from build123d import *

# Parameters (mm, degrees)
F0_W     = 20
F0_H     = 2
F1_DEPTH = 103.759
F2_R     = 2.54
F3_DEPTH = 12.7
F4_R     = 5.4
F4_R_2   = 2.54
F5_DEPTH = 1.5


with BuildPart() as f1:
    # F0 (on Right) → F1 (new body)
    with BuildSketch(Plane.YZ):
        with Locations((10, 1)):
            Rectangle(F0_W, F0_H)
    extrude(amount=F1_DEPTH)

    # F2 (on face) → F3 (cut, symmetric)
    with BuildSketch(Plane(origin=(0, 0, 0), x_dir=(1, 0, 0), z_dir=(0, 0, -1))):
        with Locations((87.503, -10)):
            Circle(F2_R)
        with Locations((16.383, -10)):
            Circle(F2_R)
        with Locations((51.943, -10)):
            Circle(F2_R)
    extrude(amount=F3_DEPTH, both=True, mode=Mode.SUBTRACT)

    # F4 (on face) → F5 (join)
    with BuildSketch(Plane.XY.offset(2)):
        with Locations((16.383, 10)):
            Circle(F4_R)
        with Locations((16.383, 10)):
            Circle(F4_R_2, mode=Mode.SUBTRACT)
        with Locations((51.943, 10)):
            Circle(F4_R)
        with Locations((51.943, 10)):
            Circle(F4_R_2, mode=Mode.SUBTRACT)
        with Locations((87.503, 10)):
            Circle(F4_R)
        with Locations((87.503, 10)):
            Circle(F4_R_2, mode=Mode.SUBTRACT)
    extrude(amount=F5_DEPTH)


solid = f1.part
Input: part model. Units: mm. Frame: model coordinates. A direction names the side the tool comes from. Round coordinates to 2 decimals unless told otherwise and drop trailing zeros. Order: outer loops, then holes, each group sorted by start corner. A loop starts at its lowest first (then second) coordinate and runs counter-clockwise, first axis right, second up.
1. Mould query, pull axis X, two halves, no side actions, for faces 1 (the face through (51, 20, 1)), 2 (the face through (51, 17, 2)), 3 (the face through (0, 10, 1)). Classes: released by +X, released by -X, zero draft, split by the parting line, or undercut.
The answers:
face 1: zero draft
face 2: undercut
face 3: released by -X
2. Pin query (flat end, axial travel): P1, Ø6, axis at x = 62.5, y = 8, coming from the +Z side; P2, Ø3, axis at x = 87.503, y = 10, coming from the -Z side. Return the tip coordinate at first contact, or that it passes through.
The answers:
P1: stops at z = 2
P2: passes through
3. Cut plane D-D, the plane x = 12. Output: boundary loops of the cut face in (y, z).
The answers:
outline: (0, 0) - (20, 0) - (20, 2) - (13.15, 2) - (13.15, 3.5) - (6.85, 3.5) - (6.85, 2) - (0, 2) - close
4. Cut plane C-C, the plane y = 18.25. Output: boundary loops of the cut face in (x, z), then the cut area to 3 significant figures.
The answers:
outline: (0, 0) - (103.76, 0) - (103.76, 2) - (0, 2) - close
area: 208 mm2
5. Cut plane A-A, the plane z = 2.8. Output: boundary loops of the cut face in (x, y), then the cut area to 3 significant figures.
The answers:
outline: circle Ø10.8 at (16.38, 10); circle Ø10.8 at (51.94, 10); circle Ø10.8 at (87.5, 10); hole circle Ø5.08 at (16.38, 10); hole circle Ø5.08 at (51.94, 10); hole circle Ø5.08 at (87.5, 10)
area: 214 mm2
6. Material intervals for line 1 (X direction, y = 10, z = 1.1); line 2 (X direction, y = 8.25, z = 2.25); line 3 (X direction, y = 14.25, z = 2.3), sorted ascending.
The answers:
line 1: x = 0 to 13.84, 18.92 to 49.4, 54.48 to 84.96, 90.04 to 103.76
line 2: x = 11.27 to 14.54, 18.22 to 21.49, 46.83 to 50.1, 53.78 to 57.05, 82.39 to 85.66, 89.34 to 92.61
line 3: x = 13.05 to 19.71, 48.61 to 55.27, 84.17 to 90.83
7. Set-up query: faces 4 (the face through (51, 14, 0)), 5 (the face through (56.93, 7.93, 2.74)). Return all of +Z, -Z, +X, -X, +Y, -Y with unobstructed straight access to the full face (end or side cutting, diameter ignored); none if empty.
The answers:
face 4: -Z, +X, -X, +Y, -Y
face 5: +Z
8. Cut plane B-B, the plane y = 10. Output: boundary loops of the cut face in (x, z), then the cut area to 3 significant figures.
The answers:
outline: (0, 0) - (13.84, 0) - (13.84, 3.5) - (10.98, 3.5) - (10.98, 2) - (0, 2) - close; (18.92, 0) - (49.4, 0) - (49.4, 3.5) - (46.54, 3.5) - (46.54, 2) - (21.78, 2) - (21.78, 3.5) - (18.92, 3.5) - close; (54.48, 0) - (84.96, 0) - (84.96, 3.5) - (82.1, 3.5) - (82.1, 2) - (57.34, 2) - (57.34, 3.5) - (54.48, 3.5) - close; (90.04, 0) - (103.76, 0) - (103.76, 2) - (92.9, 2) - (92.9, 3.5) - (90.04, 3.5) - close
area: 203 mm2
